Autodesk Fusion 360 part; units mm, degrees
sketch "Skizze1" plane through (0, 0, 0) normal (0, 0, 1) x (1, 0, 0)
  line L0 (0, 0) -> (45, 0)
  line L1 (45, 0) -> (45, 17)
  line L2 (45, 17) -> (0, 17)
  line L3 (0, 17) -> (0, 0)
  line L4 (0, 0) -> (45, 0)
  line L5 (45, 0) -> (45, 5)
  line L6 (45, 5) -> (0, 5)
  line L7 (0, 5) -> (0, 0)
  line L8 (45, 17) -> (0, 17)
  line L9 (0, 17) -> (0, 12)
  line L10 (0, 12) -> (45, 12)
  line L11 (45, 12) -> (45, 17)
  line L12 (45, 0) -> (39.2, 0)
  line L13 (39.2, 0) -> (39.2, 5.5)
  line L14 (39.2, 5.5) -> (45, 5.5)
  line L15 (45, 5.5) -> (45, 0)
  line L16 (0, 0) -> (4.9, 0)
  line L17 (4.9, 0) -> (4.9, 5.5)
  line L18 (4.9, 5.5) -> (0, 5.5)
  line L19 (0, 5.5) -> (0, 0)
  dimension "d1" = 45
  dimension "d2" = 17
  dimension "d3" = 5
  dimension "d8" = 5
  dimension "d12" = 5.8
  dimension "d13" = 5.5
  dimension "d14" = 4.9
  dimension "d15" = 5.5
extrude "Extrusion1" add sketch "Skizze1" along normal blind 25 contours L3 L6 L17 L18 L19 | L1 L3 L6 L10 L13 L14 L17 L18 | L1 L6 L13 L14 L15 | L1 L2 L3 L8 L9 L10 L11
extrude "Extrusion2" add sketch "Skizze1" along normal blind 10 contours L0 L3 L4 L6 L7 L16 L17 L19 | L0 L4 L6 L13 L17 | L0 L1 L4 L5 L6 L12 L13 L15
extrude "Extrusion3" cut sketch "Skizze1" along normal blind 10 from surface at 15 contours L1 L2 L3 L8 L9 L10 L11
sketch "Skizze2" plane through (0, 12, 0) normal (0, 1, 0) x (-1, 0, 0)
  line L0 (-45, 15) -> (0, 15)
  line L1 (0, 15) -> (0, 25)
  line L2 (0, 25) -> (-45, 25)
  line L3 (-45, 25) -> (-45, 15)
  line L4 (0, 25) -> (-5, 25)
  line L5 (-5, 25) -> (-5, 20)
  line L6 (-5, 20) -> (0, 20)
  line L7 (0, 20) -> (0, 25)
  line L8 (-45, 25) -> (-40, 25)
  line L9 (-40, 25) -> (-40, 20)
  line L10 (-40, 20) -> (-45, 20)
  line L11 (-45, 20) -> (-45, 25)
  dimension "d19" = 5
  dimension "d20" = 5
  dimension "d21" = 5
  dimension "d22" = 5
draft "Verjüngung1" angle -15 neutral plane through (45, 17, 0) pull (0, 1, 0) 1 faces at (15, 15.3333, 15)
hole "Bohrung3" at (39.2, 5.5, 0) at (4.9, 5.5, 0) direction (0, 0, 1) diameter 2.5 depth 10 tip angle 180
hole "Bohrung4" at (40, 12, 20) at (5, 12, 20) direction (0, -1, 0) diameter 3 depth 10 tip angle 180 countersink diameter 6.5 countersink angle 90
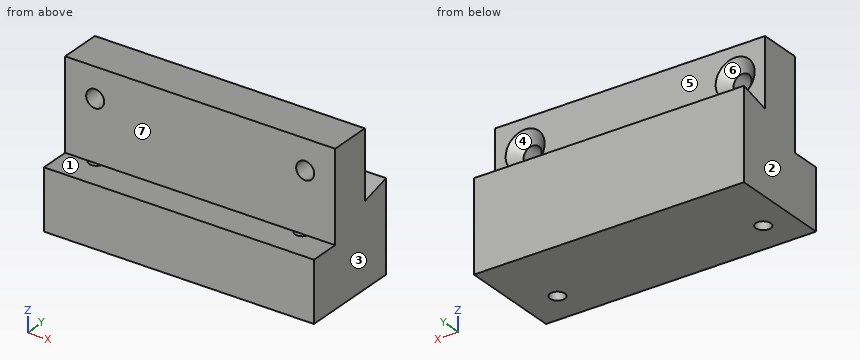
Geometry: final body of the model. Coordinates: model frame, mm. Face numbers are marked on the shaded views. A direction names the side the tool comes from. Round coordinates to 2 decimals unless told otherwise and drop trailing zeros. Loops run counter-clockwise (first coordinate to the right, second up) from the corner with the lowest first, then second, coordinate; pieces in that order, holes last.
Item 1: Mould query, pull axis X, two halves, no side actions, for the marked faces 1, 2, 3 and 4. Classes: released by +X, released by -X, zero draft, split by the parting line, or undercut.
Checked values:
face 1: zero draft
face 2: released by -X
face 3: released by +X
face 4: undercut
Item 2: Section B-B, the plane y = 11.25. Output: boundary loops of the cut face in (x, z).
Checked values:
outline: (0, 0) - (45, 0) - (45, 25) - (0, 25) - close; hole circle Ø5 at (5, 20); hole circle Ø5 at (40, 20)
Item 3: Line query: L1, parallel to X at y = 5.5, z = 2; L2, parallel to X at y = 6.8, z = 20; L3, parallel to Y at x = 4.9, z = 5. Output: solid intervals per line, ascending.
Checked values:
L1: x = 0 to 3.65, 6.15 to 37.95, 40.45 to 45
L2: x = 0 to 3.5, 6.5 to 38.5, 41.5 to 45
L3: y = 0 to 4.25, 6.75 to 17
Item 4: Section C-C, the plane x = 19.5. Output: boundary loops of the cut face in (y, z).
Checked values:
outline: (0, 0) - (17, 0) - (17, 15) - (12, 13.66) - (12, 25) - (5, 25) - (5, 10) - (0, 10) - close
Item 5: Contact query for flat-ended pins moving along their axis: P1, Ø2, axis at x = 4.9, y = 5.5, coming from the -Z side; P2, Ø6, axis at y = 5, z = 21.5, coming from the -X side; P3, Ø4.5, axis at x = 26, z = 17, coming from the -Y side; P4, Ø5.5, axis at x = 18.5, z = 22, coming from the +Y side. Output: stop coordinate, or through.
Checked values:
P1: stops at z = 10
P2: stops at x = 0
P3: stops at y = 5
P4: stops at y = 12
Item 6: Section A-A, the plane z = 20. Output: boundary loops of the cut face in (x, y).
Checked values:
outline: (0, 5) - (3.5, 5) - (3.5, 10.25) - (1.75, 12) - (0, 12) - close; (6.5, 5) - (38.5, 5) - (38.5, 10.25) - (36.75, 12) - (8.25, 12) - (6.5, 10.25) - close; (41.5, 5) - (45, 5) - (45, 12) - (43.25, 12) - (41.5, 10.25) - close
Item 7: Reachability of the marked faces 5, 6 and 7 from +Z, -Z, +X, -X, +Y, -Y: full face, straight path, thin tool, end or side. Return the list, or none.
Checked values:
face 5: +Z, +X, -X
face 6: +Y
face 7: +Z, +X, -X, -Y
Item 8: Section D-D, the plane z = 16.25. Output: boundary loops of the cut face in (x, y).
Checked values:
outline: (0, 5) - (45, 5) - (45, 12) - (0, 12) - close
